Design review of the part built by this model. Coordinates are the model's own, in mm. A direction names the side the tool comes from. Round coordinates to 2 decimals unless told otherwise and drop trailing zeros. Order: outer loops, then holes, each group sorted by start corner. A loop starts at its lowest first (then second) coordinate and runs counter-clockwise, first axis right, second up.
from build123d import *

# Parameters (mm, degrees)
F0_W     = 5.556377
F0_H     = 22.225
F1_DEPTH = 6.35
F2_W     = 3.968877
F2_H     = 20.6375
F3_DEPTH = 1.5875
F4_R     = 1.35255
F5_DEPTH = 6.35
F6_SIZE  = 3.57124


with BuildPart() as f1:
    # F0 (on Top) → F1 (new body)
    with BuildSketch(Plane.XY):
        with Locations((2.7781885, -11.1125)):
            Rectangle(F0_W, F0_H)
    extrude(amount=F1_DEPTH)

    # F2 (on face) → F3 (join)
    with BuildSketch(Plane(origin=(0, 0, 0), x_dir=(1, 0, 0), z_dir=(0, 0, -1))):
        with Locations((1.9844385, 10.31875)):
            Rectangle(F2_W, F2_H)
    extrude(amount=F3_DEPTH)

    # F4 (on face) → F5 (cut)
    with BuildSketch(Plane(origin=(0, 0, 0), x_dir=(0, -1, 0), z_dir=(-1, 0, 0))):
        with Locations((17.4625, 3.175)):
            Circle(F4_R)
        with Locations((3.175, 3.175)):
            Circle(F4_R)
    extrude(amount=-F5_DEPTH, mode=Mode.SUBTRACT)

    # F6
    f6_edges = [f1.edges().sort_by_distance(p)[0] for p in [
        (3.968877, -20.6375, -0.79375),
    ]]
    chamfer(f6_edges, length=F6_SIZE)


solid = f1.part
1) Take a section at C-C on x = 3.65. State how many separate pieces and enclosed holes the cut face has, plus the area to 3 significant figures.
Results:
separate pieces: 1
enclosed holes: 2
area: 157 mm2
2) To check wall thickness, follow line 1 along Y through (x, z) = (2.35, 3.25) (3 decimals); line 2 along Y through (x, z) = (1.8, 2.5) (3 decimals); line 3 along Z through (x, y) = (5.1, -5.25). State the ranges of each line that lie inside material, in increasing order.
Results:
line 1: y = -22.225 to -18.813, -16.112 to -4.525, -1.825 to 0
line 2: y = -22.225 to -18.635, -16.29 to -4.347, -2.003 to 0
line 3: z = 0 to 6.35
3) Take a section at B-B on y = -5.5. Give the boundary of the cut face in (x, z).
Results:
outline: (0, -1.59) - (3.97, -1.59) - (3.97, 0) - (5.56, 0) - (5.56, 6.35) - (0, 6.35) - close
4) Take a section at D-D on z = -0.25. Give the boundary of the cut face in (x, y).
Results:
outline: (0, -20.64) - (0.4, -20.64) - (3.97, -17.07) - (3.97, 0) - (0, 0) - close
5) The part is to be moulded in two halves that separate along Y. For faces 4 (the face through (3, -22.225, 3)), 5 (the face through (2.739, -3.902, 4.315)), 6 (the face through (5.556, -11, 3)), say which applies: released by +Y, released by -Y, zero draft, split by the parting line, or undercut.
Results:
face 4: released by -Y
face 5: undercut
face 6: zero draft
6) For faces 1 (the face through (3, -11, 6.35)), 2 (the face through (3.969, -8, -1)), 3 (the face through (2.208, -18.827, -0.783)), list the 3-axis set-ups (+Z, -Z, +X, -X, +Y, -Y) from which the entire face can be reached by the end or side of a thin tool; tool diameter is ignored.
Results:
face 1: +Z, +X, -X, +Y, -Y
face 2: -Z, +X, +Y, -Y
face 3: -Z, +X, -Y
7) Take a section at A-A on z = 3.75. Give the boundary of the cut face in (x, y) (3 decimals), plus the area to 3 significant figures.
Results:
outline: (0, -22.225) - (5.556, -22.225) - (5.556, -18.687) - (0, -18.687) - close; (0, -16.238) - (5.556, -16.238) - (5.556, -4.399) - (0, -4.399) - close; (0, -1.951) - (5.556, -1.951) - (5.556, 0) - (0, 0) - close
area: 96.3 mm2
